Could you check a few things on this model? Use its own coordinates, in mm. Face numbers are marked on the shaded views. A direction names the side the tool comes from. Coordinates: 2 decimals unless noted, no trailing zeros. Loops run counter-clockwise (first coordinate to the right, second up) from the corner with the lowest first, then second, coordinate; pieces in that order, holes last.
1) Imagine slicing it at A-A on x = 0. Please give me the cut outline in (y, z) (3 decimals).
2) Imagine slicing it at D-D on z = -7.5. Please give me the cut outline in (x, y), plus the area to 3 significant figures.
3) Imagine slicing it at C-C on y = -7.75. Please give me the cut outline in (x, z) (1 decimal).
4) Imagine slicing it at B-B on z = 0. Please give me the cut outline in (x, y).
5) Will these pins go through, and if not, where does the flat tip stop? P1, Ø8, axis at y = -7.5, z = -11.5, coming from the -X side; P2, Ø5, axis at y = -1.5, z = -18, coming from the -X side; P3, Ø1.5, axis at x = -16, y = 4, coming from the -Z side; P4, Ø1.5, axis at y = -0.5, z = 9, coming from the +X side.
6) If I drill on line 1 along Y through (x, z) = (12, 20.5); line 2 along Z through (x, y) = (-19, -4); line 3 along X through (y, z) = (-8, 13), over which ranges is the centre line in solid material (lowest first)?
7) Thinking about a two-plate mould opening in X: for the marked faces 3, 4, 5 and 6, which applies, released by +X, released by -X, zero draft, split by the parting line, or undercut?
8) For the marked faces 1 and 2, which set-ups out of +Z, -Z, +X, -X, +Y, -Y let a thin tool reach every point of the face, with its end or its side?
```python
from build123d import *

# Parameters (mm, degrees)
SKETCH2_R           = 27
BOSS_EXTRUDE1_DEPTH = 6
SKETCH1_R           = 3.4
BOSS_EXTRUDE2_DEPTH = 9
CHAMFER1_SIZE       = 1


with BuildPart() as part:
    # Sketch2 → Boss-Extrude1 (new body)
    with BuildSketch(Plane(origin=(0, 0, 0), x_dir=(1, 0, 0), z_dir=(0, 1, 0))):
        with Locations(Location((0, 0, 0), (0, 0, 270))):
            Circle(SKETCH2_R)
    extrude(amount=BOSS_EXTRUDE1_DEPTH)

    # Sketch1 → Boss-Extrude2 (add)
    with BuildSketch(Plane(origin=(0, 0, 0), x_dir=(1, 0, 0), z_dir=(0, 1, 0))):
        with Locations(Location((0, 21.875, 0), (0, 0, 270))):
            Circle(SKETCH1_R)
        with Locations(Location((18.944305708, -10.9375, 0), (0, 0, 270))):
            Circle(SKETCH1_R)
        with Locations(Location((-18.944305708, -10.9375, 0), (0, 0, 270))):
            Circle(SKETCH1_R)
    extrude(amount=-BOSS_EXTRUDE2_DEPTH)

    # Chamfer1
    chamfer1_edges = [part.edges().sort_by_distance(p)[0] for p in [
        (-18.944305708, 0, 7.5375),
        (18.944305708, 0, 7.5375),
        (0, 0, -25.275),
    ]]
    chamfer(chamfer1_edges, length=CHAMFER1_SIZE)


solid = part.part
```
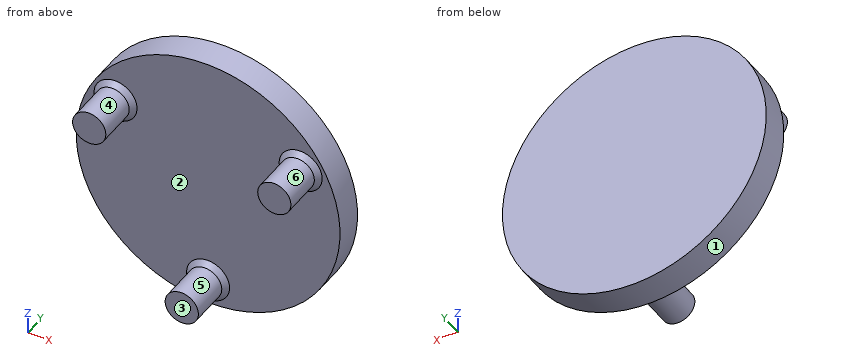
Filled in:
1. outline: (-9, -25.275) - (-1, -25.275) - (0, -26.275) - (0, -27) - (6, -27) - (6, 27) - (0, 27) - (0, -17.475) - (-1, -18.475) - (-9, -18.475) - close
2. outline: (-25.94, 0) - (25.94, 0) - (25.94, 6) - (-25.94, 6) - close
2. area: 311 mm2
3. outline: circle Ø6.8 at (-18.9, 10.9); circle Ø6.8 at (0, -21.9); circle Ø6.8 at (18.9, 10.9)
4. outline: (-27, 0) - (27, 0) - (27, 6) - (-27, 6) - close
5. P1: passes through
5. P2: stops at x = -21.75
5. P3: stops at z = -22.28
5. P4: stops at x = 25.65
6. line 1: y = 0 to 6
6. line 2: z = 7.54 to 14.34
6. line 3: x = -21.65 to -16.24, 16.24 to 21.65
7. face 3: zero draft
7. face 4: undercut
7. face 5: split by the parting line
7. face 6: undercut
8. face 1: +Y, -Y
8. face 2: -Y
